Design review of the part built by this model. Coordinates are the model's own, in mm. Face numbers are marked on the shaded views. Give positions to 0.01 mm unless a question says otherwise; leave off trailing zeros. Write each loop counter-clockwise with the first axis right and the second up, starting at its lowest first coordinate (ties: lowest second). Pieces come first, ordered by that corner, then holes. Notation, with made-up numbers: M 9.5,68.5 L 36.5,68.5 A36 ccw 36.5,104.5 Z; hole C 57,-18 d1. An arc over 180 degrees is marked long. Use a Markdown table: item, result. Add a question column.
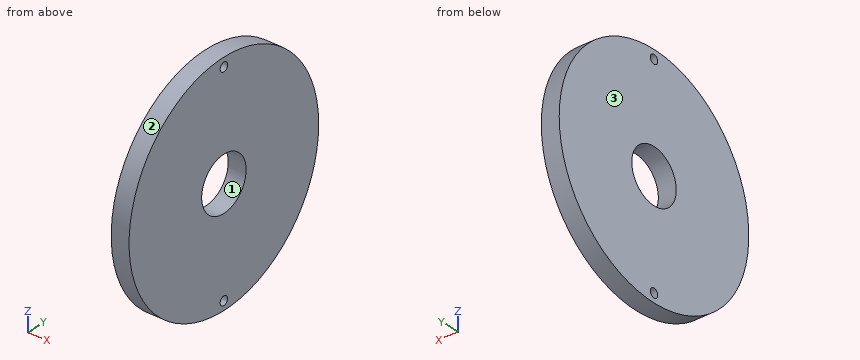
```python
from build123d import *

# Parameters (mm, degrees)
F0_R     = 40.64
F1_DEPTH = 6.35
F2_R     = 1.5875
F3_DEPTH = 6.35
F4_R     = 9.525
F5_DEPTH = 6.35


with BuildPart() as f1:
    # F0 (on Right) → F1 (new body)
    with BuildSketch(Plane.YZ):
        Circle(F0_R)
    extrude(amount=F1_DEPTH)

    # F2 (on face) → F3 (cut)
    with BuildSketch(Plane.YZ.offset(6.35)):
        with Locations((0, 37.465)):
            Circle(F2_R)
        with Locations((0, -37.465)):
            Circle(F2_R)
    extrude(amount=-F3_DEPTH, mode=Mode.SUBTRACT)

    # F4 (on face) → F5 (cut)
    with BuildSketch(Plane.YZ.offset(6.35)):
        Circle(F4_R)
    extrude(amount=-F5_DEPTH, mode=Mode.SUBTRACT)


solid = f1.part
```
(1) The part is to be moulded in two halves that separate along Z. For the marked faces 1, 2 and 3, say which applies: released by +Z, released by -Z, zero draft, split by the parting line, or undercut.
(2) Add section A-A on z = 0. Give the boundary of the cut face in (x, y) (3 decimals), then the cut area to 3 significant figures.
(3) For pin 1 (3 mm diameter, centred on x = 2, y = 23, fed in from -Z); pin 2 (1.9 mm diameter, centred on y = 0, z = -37.465, fed in from -X), all flat-tipped, find the tip position at first contact; note any pin that passes through.
(4) Add section B-B on y = 0. Give the number of separate pieces and of enclosed holes in the cut face, then the cut area to 3 significant figures.
(5) Add section D-D on z = -21.5. Give the boundary of the cut face in (x, y).
(6) Wall thickness on L1, parallel to Z at x = 2.5, y = 0 (1 decimal); L2, parallel to Z at x = 3.5, y = 1; L3, parallel to Z at x = 6, y = 5: over which ranges is each line inside the solid? List them lowest first.
From the geometry:
| question | item | result |
|---|---|---|
| 1 | face 1 | undercut |
| 1 | face 2 | split by the parting line |
| 1 | face 3 | zero draft |
| 2 | outline | M 0,-40.64 L 6.35,-40.64 L 6.35,-9.525 L 0,-9.525 Z; M 0,9.525 L 6.35,9.525 L 6.35,40.64 L 0,40.64 Z |
| 2 | area | 395 mm^2 |
| 3 | pin 1 | stops at z = -34.49 |
| 3 | pin 2 | passes through |
| 4 | separate pieces | 4 |
| 4 | enclosed holes | 0 |
| 4 | area | 355 mm^2 |
| 5 | outline | M 0,-34.49 L 6.35,-34.49 L 6.35,34.49 L 0,34.49 Z |
| 6 | L1 | z = -40.6 to -39.1, -35.9 to -9.5, 9.5 to 35.9, 39.1 to 40.6 |
| 6 | L2 | z = -40.63 to -38.7, -36.23 to -9.47, 9.47 to 36.23, 38.7 to 40.63 |
| 6 | L3 | z = -40.33 to -8.11, 8.11 to 40.33 |
